Could you check a few things on this model? Use its own coordinates, in mm. A direction names the side the tool comes from. Round coordinates to 2 decimals unless told otherwise and drop trailing zeros. Write each loop counter-clockwise with the first axis right and the second up, starting at its lowest first coordinate (ties: lowest second). Pieces come first, ordered by that corner, then holes. Notation, with made-up numbers: (-39.5, 32.25) - (2.5, 32.25) arc R16 cw to (2.5, 40.25) - close; hole circle Ø4 at (89, -32). An arc over 180 degrees is marked (long way). Write each question's results on one line, items separated by ' | '. Start each with the question number.
(1) On a 3-axis mill with a long thin cutter (end or side, diameter ignored), from which of +Z, -Z, +X, -X, +Y, -Y can I reach the whole of each face in a straight line? I mean faces 4 (the flat face through (-1.5, -31, 2)), 5 (the flat face through (-2, -64, 0)). Say none if no direction works.
(2) For P1, Ø3, axis at x = 3.5, z = 3.5, coming from the -Y side, with a flat end and sliding along its axis, tell me the tip position at first contact or that it passes through.
(3) Thinking about a two-plate mould opening in Y: for faces 1 (the flat face through (5, -64, 2)), 2 (the cylindrical face through (0, -105, 2)), 3 (the cylindrical face through (0, -51.5, 2.5)), which applies, +Y half, -Y half, draft (parallel to the pull), parting line (faces both ways), or undercut?
(4) Imagine slicing it at A-A on z = 0.8. State how many separate pieces and enclosed holes the cut face has, then the cut area to 3 significant figures.
(5) Please list where these lines run through material, in increasing order: line 1 (Y direction, x = 0, z = 1.3); line 2 (X direction, y = -65, z = 3.05); line 3 (Y direction, x = -0.5, z = 0.8). Write a range as [from, to].
(6) Imagine slicing it at D-D on x = -3.25. Write out the boundary of the cut face in (y, z), then the cut area to 3 significant figures.
(7) Imagine slicing it at C-C on x = 0.5. Write out the boundary of the cut face in (y, z), then the cut area to 3 significant figures.
(8) Imagine slicing it at B-B on y = -65. Write out the boundary of the cut face in (x, z), then the cut area to 3 significant figures.
```python
from build123d import *

# Parameters (mm, degrees)
CROQUIS1_R              = 1.5
SALIENTE_EXTRUIR1_DEPTH = 5
CORTAR_EXTRUIR1_START   = -10
CORTAR_EXTRUIR1_DEPTH   = 10
CROQUIS9_W              = 21.716341412
CROQUIS9_H              = 41.96907492
CORTAR_EXTRUIR2_DEPTH   = 10
SALIENTE_EXTRUIR2_DEPTH = 5
SALIENTE_EXTRUIR3_DEPTH = 5


with BuildPart() as part:
    # Croquis1 → Saliente-Extruir1 (new body)
    with BuildSketch(Plane.XY):
        with BuildLine():
            Line((5, 0), (5, -100))
            ThreePointArc((5, -100), (0, -105), (-5, -100))
            Line((-5, -100), (-5, 0))
            ThreePointArc((-5, 0), (0, 5), (5, 0))
        make_face()
        Circle(CROQUIS1_R, mode=Mode.SUBTRACT)
        with Locations((0, -100)):
            Circle(CROQUIS1_R, mode=Mode.SUBTRACT)
        with Locations((0, -65)):
            Circle(CROQUIS1_R, mode=Mode.SUBTRACT)
    extrude(amount=SALIENTE_EXTRUIR1_DEPTH)

    # Croquis8 → Cortar-Extruir1 (cut)
    with BuildSketch(Plane.XY.offset(5).offset(CORTAR_EXTRUIR1_START)):
        with BuildLine():
            Line((1.5, 0), (1.5, -50))
            ThreePointArc((1.5, -50), (0, -51.5), (-1.5, -50))
            Line((-1.5, -50), (-1.5, 0))
            ThreePointArc((-1.5, 0), (0, 1.5), (1.5, 0))
        make_face()
    extrude(amount=CORTAR_EXTRUIR1_DEPTH, mode=Mode.SUBTRACT)

    # Croquis9 → Cortar-Extruir2 (cut)
    with BuildSketch(Plane.XY.offset(5)):
        with Locations((5.858170706, -8.775938245)):
            Rectangle(CROQUIS9_W, CROQUIS9_H)
    extrude(amount=-CORTAR_EXTRUIR2_DEPTH, mode=Mode.SUBTRACT)



with BuildPart() as body_2:
    # Croquis10 → Saliente-Extruir2 (new body)
    with BuildSketch(Plane.XY.offset(5)):
        with BuildLine():
            Line((1.5, -29.760475705), (5, -29.760475705))
            ThreePointArc((5, -29.760475705), (0.000823646, -24.758830917), (-4.999998466, -29.758830217))
            Line((-4.999998466, -29.758830217), (-1.499999097, -29.758830217))
            ThreePointArc((-1.499999097, -29.758830217), (0.000823646, -28.258830443), (1.5, -29.760475705))
        make_face()
    extrude(amount=-SALIENTE_EXTRUIR2_DEPTH)


with BuildPart() as part_1:
    add(part.part)

    add(body_2.part)  # Saliente-Extruir3 merges body 2
    # Croquis11 → Saliente-Extruir3 (add)
    with BuildSketch(Plane(origin=(0, 0, 0), x_dir=(-1, 0, 0), z_dir=(0, 0, -1))):
        with BuildLine():
            Line((-5, -29.760475705), (-5, -32.237958703))
            Line((-5, -32.237958703), (-1.5, -32.237958703))
            Line((-1.5, -32.237958703), (-1.5, -29.760475705))
            ThreePointArc((-1.5, -29.760475705), (-0.000823646, -28.258830443), (1.499999097, -29.758830217))
            Line((1.499999097, -29.758830217), (1.499999097, -32.237958703))
            Line((1.499999097, -32.237958703), (5, -32.237958703))
            Line((5, -32.237958703), (4.999998466, -29.758830217))
            ThreePointArc((4.999998466, -29.758830217), (-0.000823646, -24.758830917), (-5, -29.760475705))
        make_face()
    extrude(amount=-SALIENTE_EXTRUIR3_DEPTH)


solid = part_1.part
```
Response:
1) face 4: +Z, -Z | face 5: -Z, +X, -X, +Y, -Y
2) P1: y = -104.58
3) face 1: draft | face 2: -Y half | face 3: undercut
4) separate pieces: 1 | enclosed holes: 3 | area: 699 mm²
5) line 1: [-105, -101.5], [-98.5, -66.5], [-63.5, -51.5], [-28.26, -24.76] | line 2: [-5, -1.5], [1.5, 5] | line 3: [-104.97, -101.41], [-98.59, -66.41], [-63.59, -51.41], [-28.34, -24.78]
6) outline: (-103.8, 0) - (-25.96, 0) - (-25.96, 5) - (-103.8, 5) - close | area: 389 mm²
7) outline: (-104.97, 0) - (-101.41, 0) - (-101.41, 5) - (-104.97, 5) - close; (-98.59, 0) - (-66.41, 0) - (-66.41, 5) - (-98.59, 5) - close; (-63.59, 0) - (-51.41, 0) - (-51.41, 5) - (-63.59, 5) - close; (-28.34, 0) - (-24.78, 0) - (-24.78, 5) - (-28.34, 5) - close | area: 257 mm²
8) outline: (-5, 0) - (-1.5, 0) - (-1.5, 5) - (-5, 5) - close; (1.5, 0) - (5, 0) - (5, 5) - (1.5, 5) - close | area: 35.0 mm²
